Autodesk Inventor part; units mm, degrees
ref_plane "YZ Plane" through (0, 0, 0) normal (1, 0, 0) x (0, 1, 0)
ref_plane "XZ Plane" through (0, 0, 0) normal (0, 1, 0) x (-1, 0, 0)
ref_plane "XY Plane" through (0, 0, 0) normal (0, 0, 1) x (1, 0, 0)
sketch "Sketch1" plane through (0, 0, 0) normal (1, 0, 0) x (0, 1, 0)
  line L0 (-275, 24.5536) -> (275, 24.5536)
  line L1 (275, 24.5536) -> (275, -24.5536)
  line L2 (275, -24.5536) -> (-275, -24.5536)
  line L3 (-275, -24.5536) -> (-275, 24.5536)
  point P0 (0, 0)
  dimension "d15" = 550
extrude "Extrusion1" add sketch "Sketch1" along normal mid plane 50
sketch "Sketch2" plane through (-25, 275, 24.5536) normal (0, 1, 0) x (1, 0, 0)
  line L0 (50, 49.1071) -> (50, 0)
  line L1 (50, 4.1071) -> (5, 4.1071)
  line L2 (5, 4.1071) -> (5, 49.1071)
  line L3 (50, 49.1071) -> (0, 49.1071)
  line L4 (5, 49.1071) -> (50, 49.1071)
  line L5 (50, 49.1071) -> (50, 4.1071)
  point P0 (25, 24.5536)
extrude "Extrusion2" cut sketch "Sketch2" against normal through all
sketch "Sketch5" plane through (-25, 0, 0) normal (-1, 0, 0) x (0, 0, 1)
  line L0 (-24.5536, 275) -> (-24.5536, -275)
  line L1 (20.4464, -275) -> (20.4464, 275)
  line L2 (-24.5536, 275) -> (20.4464, 275)
  line L3 (20.4464, 275) -> (20.4464, 225)
  line L4 (20.4464, 225) -> (-24.5536, 225)
  line L5 (-24.5536, 225) -> (-24.5536, 275)
  line L6 (-24.5536, -275) -> (24.5536, -275)
  line L7 (-24.5536, -275) -> (20.4464, -275)
  line L8 (20.4464, -275) -> (20.4464, -225)
  line L9 (20.4464, -225) -> (-24.5536, -225)
  line L10 (-24.5536, -225) -> (-24.5536, -275)
  point P0 (0, 0)
extrude "Extrusion5" cut sketch "Sketch5" against normal blind 10 contours L2 L1 L4 L0 | L9 L1 L6 L0
sketch "Sketch6" plane through (-25, -275, 24.5536) normal (0, 0, 1) x (1, 0, 0)
  line L0 (0, 500) -> (0, 50)
  line L1 (50, 0) -> (50, 550)
  line L2 (0, 500) -> (50, 550)
  line L3 (50, 550) -> (0, 550)
  line L4 (0, 550) -> (0, 500)
  line L5 (0, 50) -> (50, 0)
  line L6 (0, 0) -> (50, 0)
  line L7 (50, 0) -> (0, 0)
  line L8 (0, 0) -> (0, 50)
  point P0 (25, 275)
extrude "Extrusion6" cut sketch "Sketch6" against normal blind 5 contours L4 L3 L2 | L5 L6 L8
properties part number "angle3"
Geometry check sheet. Reference: the model listing, model coordinates, mm. A direction names the side the tool comes from. Round coordinates to 2 decimals unless told otherwise and drop trailing zeros. Write each loop counter-clockwise with the first axis right and the second up, starting at its lowest first coordinate (ties: lowest second). Pieces come first, ordered by that corner, then holes. Notation, with made-up numbers: (15.25, 70.5) - (63.25, 70.5) arc R24 ccw to (63.25, 100.5) - close; hole circle Ø9 at (10, -16.75). An arc over 180 degrees is marked (long way). One line per item, written item: value.
1. Depth check by flat-ended pin: pin 1 Ø5.5 at (x, z) = (-23, 4.5) entering from -Y; pin 2 Ø8 at (x, z) = (-16.5, 4.5) entering from +Y; pin 3 Ø5 at (x, y) = (6.5, -131) entering from -Z. Enter the tip coordinate at first touch or a pass-through.
The answers:
pin 1: stops at y = -225
pin 2: stops at y = 225
pin 3: stops at z = 20.45
2. Cross-section at C-C on z = -14.5. Record the boundary of the cut face in (x, y), and give its area (3 significant figures).
The answers:
outline: (-25, -225) - (-20, -225) - (-20, 225) - (-25, 225) - close
area: 2,250 mm^2
3. Cross-section at B-B on y = 17.5. Record the boundary of the cut face in (x, z), and give its area (3 significant figures).
The answers:
outline: (-25, -24.55) - (-20, -24.55) - (-20, 20.45) - (25, 20.45) - (25, 24.55) - (-25, 24.55) - close
area: 430 mm^2
4. Set-up check for faces 1 (the face through (-25, -3, 0)), 2 (the face through (-20, 3, -2)): record each of +Z, -Z, +X, -X, +Y, -Y from which the full face is reachable in a straight line by a thin tool's end or side.
The answers:
face 1: +Z, -Z, -X, +Y, -Y
face 2: -Z, +X, +Y, -Y
5. Scan lines: L1, parallel to Z at x = -17.5, y = 177; L2, parallel to X at y = 46, z = -11; L3, parallel to Y at x = -21.5, z = 4. Record each from-to range of solid material in increasing order.
The answers:
L1: z = 20.45 to 24.55
L2: x = -25 to -20
L3: y = -225 to 225
6. Cross-section at A-A on x = -0.5. Record the boundary of the cut face in (y, z), and give its area (3 significant figures).
The answers:
outline: (-249.5, 20.45) - (249.5, 20.45) - (249.5, 24.55) - (-249.5, 24.55) - close
area: 2,050 mm^2
